from build123d import *

# Parameters (mm, degrees)
Y_KSEKLIK_EKSTR_ZYON1_DEPTH = 8
IZIM2_R                     = 1.5
KES_EKSTR_ZYON1_DEPTH       = 10
Y_KSEKLIK_EKSTR_ZYON2_DEPTH = 5


with BuildPart() as part:
    # Çizim1 → Yükseklik-Ekstrüzyon1 (new body, symmetric)
    with BuildSketch(Plane.XY):
        Polygon((-15, 27.75), (-13, 27.75), (-13, 29.75), (-13, 47.75), (-15, 47.75), (-15, 29.75), (-25, 29.75), (-25, -29.75), (-15, -29.75), (-15, -47.75), (-13, -47.75), (-13, -29.75), (-13, -27.75), (-15, -27.75), (-23, -27.75), (-23, 0), (-23, 27.75), align=None)
    extrude(amount=Y_KSEKLIK_EKSTR_ZYON1_DEPTH, both=True)

    # Çizim2 → Kes-Ekstrüzyon1 (cut)
    with BuildSketch(Plane.ZY.offset(15)):
        with Locations((0, 37.75)):
            Circle(IZIM2_R)
        with Locations((0, -37.75)):
            Circle(IZIM2_R)
    extrude(amount=-KES_EKSTR_ZYON1_DEPTH, mode=Mode.SUBTRACT)

    # Çizim4 → Yükseklik-Ekstrüzyon2 (add, symmetric)
    with BuildSketch(Plane.XY):
        Polygon((-25, 10), (-32, 10), (-32, -10), (-25, -10), (-25, -12), (-34, -12), (-34, 12), (-25, 12), align=None)
    extrude(amount=Y_KSEKLIK_EKSTR_ZYON2_DEPTH, both=True)


solid = part.part
The model under review builds one solid part; all positions refer to its coordinate system, in mm. A direction names the side the tool comes from. Round coordinates to 2 decimals unless told otherwise and drop trailing zeros. Write each loop counter-clockwise with the first axis right and the second up, starting at its lowest first coordinate (ties: lowest second). Pieces come first, ordered by that corner, then holes. Notation, with made-up numbers: (19.25, 26) - (24.25, 26) arc R15 ccw to (24.25, 40) - close; hole circle Ø8 at (38, 38). An arc over 180 degrees is marked (long way). One line per item, written item: value. Start each with the question number.
1. Consider section B-B on y = -6. Write out the cut boundary in (x, z).
2. To check wall thickness, follow L1, parallel to Y at x = -14.5, z = 0; L2, parallel to Y at x = -16.75, z = 1.75; L3, parallel to Y at x = -27.75, z = -1.5. State the ranges of each line that lie inside material, in increasing order. Write a range as from..to.
3. Consider section C-C on x = -30.25. Write out the cut boundary in (y, z).
4. Machinability: for faces 1 (the face through (-20, -29.75, 0)), 2 (the face through (-32, 0, 0)), 3 (the face through (-15, 39, 2)), 4 (the face through (-18, -27.75, 0)), which of the approach directions +Z, -Z, +X, -X, +Y, -Y give a long, thin tool a straight path to every point of the face, cutting with its end or side? Answer none if there is none.
5. The part is to be moulded in two halves that separate along Y. For faces 5 (the face through (-13, 38, 2)), 6 (the face through (-14, -47.75, 0)), 7 (the face through (-18, 27.75, 0)), say which applies: released by +Y, released by -Y, zero draft, split by the parting line, or undercut.
6. Clearance check with flat-ended pins moving along their axes: P1, Ø5, axis at y = 41.5, z = 0, coming from the -X side; P2, Ø3, axis at x = -20, z = 0.5, coming from the -Y side; P3, Ø6, axis at x = -26, z = 0, coming from the +Y side; P4, Ø2.5, axis at y = -37.75, z = 0, coming from the -X side. State where each tip first meets the part, or that it passes through.
7. Consider section A-A on z = 0. Write out the cut boundary in (x, y), and give its area (3 significant figures).
8. Consider section D-D on z = -7. Write out the cut boundary in (x, y), and give its area (3 significant figures).
Checks:
1. outline: (-34, -5) - (-32, -5) - (-32, 5) - (-34, 5) - close; (-25, -8) - (-23, -8) - (-23, 8) - (-25, 8) - close
2. L1: y = -47.75..-39.25, -36.25..-27.75, 27.75..36.25, 39.25..47.75
2. L2: y = -29.75..-27.75, 27.75..29.75
2. L3: y = -12..-10, 10..12
3. outline: (-12, -5) - (-10, -5) - (-10, 5) - (-12, 5) - close; (10, -5) - (12, -5) - (12, 5) - (10, 5) - close
4. face 1: +Z, -Z, -X, -Y
4. face 2: +Z, -Z
4. face 3: +Z, -Z, -X, +Y
4. face 4: +Z, -Z, +X
5. face 5: zero draft
5. face 6: released by -Y
5. face 7: undercut
6. P1: stops at x = -15
6. P2: stops at y = -29.75
6. P3: stops at y = 29.75
6. P4: passes through
7. outline: (-34, -12) - (-25, -12) - (-25, -29.75) - (-15, -29.75) - (-15, -36.25) - (-13, -36.25) - (-13, -27.75) - (-23, -27.75) - (-23, 27.75) - (-13, 27.75) - (-13, 36.25) - (-15, 36.25) - (-15, 29.75) - (-25, 29.75) - (-25, 12) - (-34, 12) - close; (-15, -47.75) - (-13, -47.75) - (-13, -39.25) - (-15, -39.25) - close; (-15, 39.25) - (-13, 39.25) - (-13, 47.75) - (-15, 47.75) - close; hole (-32, -10) - (-25, -10) - (-25, 10) - (-32, 10) - close
7. area: 295 mm^2
8. outline: (-25, -29.75) - (-15, -29.75) - (-15, -47.75) - (-13, -47.75) - (-13, -27.75) - (-23, -27.75) - (-23, 27.75) - (-13, 27.75) - (-13, 47.75) - (-15, 47.75) - (-15, 29.75) - (-25, 29.75) - close
8. area: 231 mm^2
